Check sheet for the drawn part. Datum: minimum x, y, z corner. Units: mm. A direction names the side the tool comes from. Round coordinates to 2 decimals unless told otherwise and drop trailing zeros. Write each loop counter-clockwise with the first axis right and the second up, starting at its lowest first coordinate (ties: lowest second). Pieces come first, ordered by that corner, then holes.
Item 1: Material ranges on line 1 (Y direction, x = 32, z = 8); line 2 (X direction, y = 32, z = 4); line 3 (Z direction, x = 167, y = 41.5), recorded low to high.
Item 2: Tool access check on the marked faces 1, 2, 3, 4 and 5. Record the directions out of +Z, -Z, +X, -X, +Y, -Y that give a thin tool (end or side, any length) a straight path to the whole face; none if there is none.
Item 3: Release check for a two-part mould opening along X. For the marked faces 6, 7 and 8 record: +X half, -X half, draft (parallel to the pull), parting line (faces both ways), or undercut.
Item 4: Cross-section at C-C on z = 28. Enter the section's corners in (x, y).
Item 5: Cross-section at D-D on y = 5. Enter the section's corners in (x, z), plus the area to 3 significant figures.
Item 6: Cross-section at A-A on z = 14. Enter the section's corners in (x, y).
Item 7: Go/stop test with flat-tipped pins: pin 1 Ø3 at (y, z) = (36.5, 46.5) entering from +X; pin 2 Ø5 at (y, z) = (24.5, 8) entering from +X; pin 3 Ø10 at (y, z) = (16.5, 45.5) entering from -X. Record where each tip stops, or that it passes through.
Item 8: Cross-section at B-B on y = 38. Enter the section's corners in (x, z).
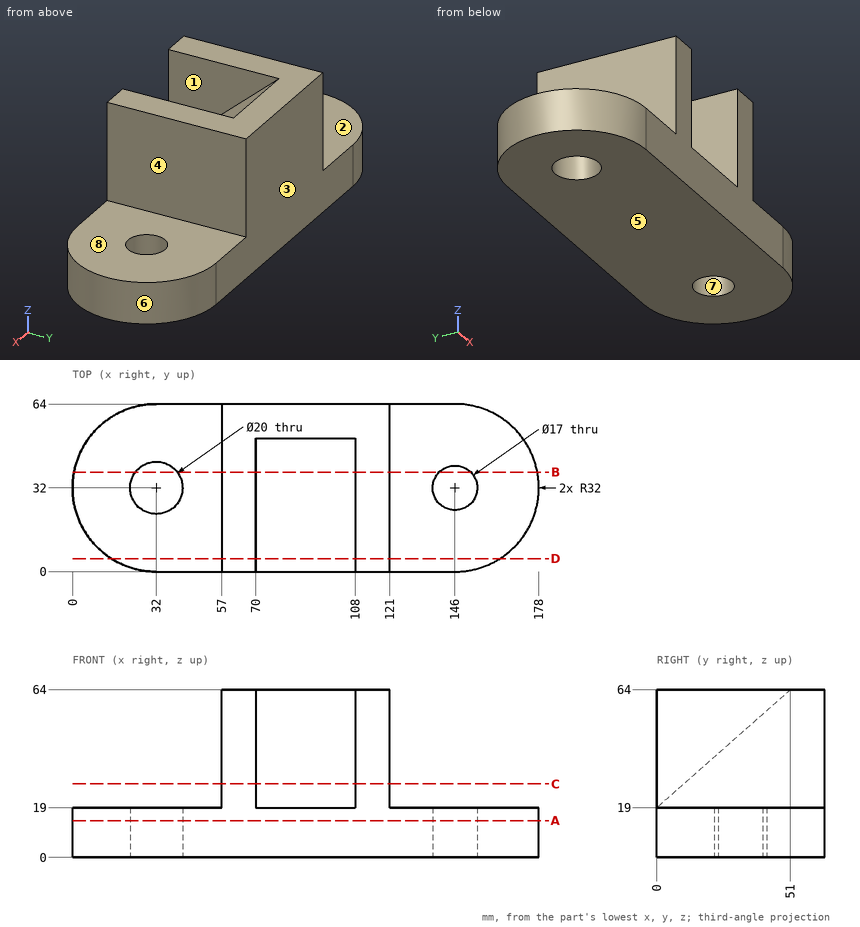
Response values:
1. line 1: y = 0 to 22, 42 to 64
1. line 2: x = 0 to 22, 42 to 137.5, 154.5 to 178
1. line 3: z = 0 to 19
2. face 1: +Z, -Y
2. face 2: +Z, -X, +Y, -Y
2. face 3: +Z, -Z, +X, -X, +Y
2. face 4: +Z, +X, +Y, -Y
2. face 5: -Z, +X, -X, +Y, -Y
3. face 6: +X half
3. face 7: undercut
3. face 8: draft
4. outline: (57, 0) - (70, 0) - (70, 10.2) - (108, 10.2) - (108, 0) - (121, 0) - (121, 64) - (57, 64) - close
5. outline: (14.82, 0) - (163.18, 0) - (163.18, 19) - (121, 19) - (121, 64) - (108, 64) - (108, 23.41) - (70, 23.41) - (70, 64) - (57, 64) - (57, 19) - (14.82, 19) - close
5. area: 4,160 mm2
6. outline: (32, 0) - (146, 0) arc R32 ccw to (146, 64) - (32, 64) arc R32 ccw to start; hole circle Ø20 at (32, 32); hole circle Ø17 at (146, 32)
7. pin 1: stops at x = 121
7. pin 2: stops at x = 177.61
7. pin 3: stops at x = 57
8. outline: (0.57, 0) - (24, 0) - (24, 19) - (0.57, 19) - close; (40, 0) - (139.98, 0) - (139.98, 19) - (121, 19) - (121, 64) - (108, 64) - (108, 52.53) - (70, 52.53) - (70, 64) - (57, 64) - (57, 19) - (40, 19) - close; (152.02, 0) - (177.43, 0) - (177.43, 19) - (152.02, 19) - close
